from build123d import *

# Parameters (mm, degrees)
SKETCH2_W                                     = 609.6
SKETCH2_H                                     = 914.4
BOSS_EXTRUDE1_DEPTH                           = 25.4
F_1_4_20_TAPPED_HOLE1_D                       = 5.1054
SKETCH46_R                                    = 76.2
CUT_EXTRUDE3_DEPTH                            = 26.4
SKETCH47_R                                    = 50.8
CUT_EXTRUDE4_DEPTH                            = 26.4
CBORE_FOR_1_4_SOCKET_HEAD_CAP_SCREW1_AT_COUNT = 2
CBORE_FOR_1_4_SOCKET_HEAD_CAP_SCREW1_AT_PITCH = 558.8
CBORE_FOR_1_4_SOCKET_HEAD_CAP_SCREW1_2_COUNT  = 2
CBORE_FOR_1_4_SOCKET_HEAD_CAP_SCREW1_2_PITCH  = 1028.621601951
CBORE_FOR_1_4_SOCKET_HEAD_CAP_SCREW1_3_COUNT  = 2
CBORE_FOR_1_4_SOCKET_HEAD_CAP_SCREW1_3_PITCH  = 863.6
CBORE_FOR_1_4_SOCKET_HEAD_CAP_SCREW1_4_COUNT  = 2
CBORE_FOR_1_4_SOCKET_HEAD_CAP_SCREW1_4_PITCH  = 523.634414453
CBORE_FOR_1_4_SOCKET_HEAD_CAP_SCREW1_5_COUNT  = 2
CBORE_FOR_1_4_SOCKET_HEAD_CAP_SCREW1_5_PITCH  = 579.765780294
CBORE_FOR_1_4_SOCKET_HEAD_CAP_SCREW1_6_COUNT  = 2
CBORE_FOR_1_4_SOCKET_HEAD_CAP_SCREW1_6_PITCH  = 452.234142895
CBORE_FOR_1_4_SOCKET_HEAD_CAP_SCREW1_7_COUNT  = 2
CBORE_FOR_1_4_SOCKET_HEAD_CAP_SCREW1_7_PITCH  = 377.598146182


with BuildPart() as part:
    # Sketch2 → Boss-Extrude1 (new body)
    with BuildSketch(Plane(origin=(0, 0, 0), x_dir=(1, 0, 0), z_dir=(0, 1, 0))):
        with Locations((659.0884662, -7.96825605)):
            Rectangle(SKETCH2_W, SKETCH2_H)
    extrude(amount=BOSS_EXTRUDE1_DEPTH)

    # 1/4-20 Tapped Hole1 (through all)
    with Locations(Plane(origin=(0, 25.4, 0), x_dir=(1, 0, 0), z_dir=(0, 1, 0))):
        with Locations((366.9884662, 436.53174395)):
            Hole(F_1_4_20_TAPPED_HOLE1_D / 2)

    # Sketch46 → Cut-Extrude3 (cut, through all)
    with BuildSketch(Plane(origin=(0, 25.4, 0), x_dir=(1, 0, 0), z_dir=(0, 1, 0))):
        with Locations((786.0884662, -261.96825605)):
            Circle(SKETCH46_R)
    extrude(amount=-CUT_EXTRUDE3_DEPTH, mode=Mode.SUBTRACT)

    # Sketch47 → Cut-Extrude4 (cut, through all)
    with BuildSketch(Plane(origin=(0, 25.4, 0), x_dir=(1, 0, 0), z_dir=(0, 1, 0))):
        with Locations((582.8884662, -7.96825605)):
            Circle(SKETCH47_R)
    extrude(amount=-CUT_EXTRUDE4_DEPTH, mode=Mode.SUBTRACT)

    # Sketch51 → CBORE for 1/4 Socket Head Cap Screw1 (revolve, cut)
    with BuildSketch(Plane(origin=(379.6884662, 25.4, -423.83174395), x_dir=(0, 0, 1), z_dir=(1, 0, 0))):
        Polygon((0, 0), (0, 25.4), (3.3782, 25.4), (3.3782, 6.35), (5.55625, 6.35), (5.55625, 0.635), (6.19125, 0), align=None)
    cbore_for_1_4_socket_head_cap_screw1 = revolve(axis=Axis((379.6884662, 31.75, -423.83174395), (0, -1, 0)), mode=Mode.SUBTRACT)

    # CBORE for 1/4 Socket Head Cap Screw1 at: CBORE for 1/4 Socket Head Cap Screw1 ×2
    with Locations(*[(i * CBORE_FOR_1_4_SOCKET_HEAD_CAP_SCREW1_AT_PITCH, 0, 0) for i in range(1, CBORE_FOR_1_4_SOCKET_HEAD_CAP_SCREW1_AT_COUNT)]):
        add(cbore_for_1_4_socket_head_cap_screw1, mode=Mode.SUBTRACT)

    # CBORE for 1_4 Socket Head Cap Screw1 2: CBORE for 1/4 Socket Head Cap Screw1 ×2
    with Locations(*[Vector(0.543251278, 0, 0.839570157) * (i * CBORE_FOR_1_4_SOCKET_HEAD_CAP_SCREW1_2_PITCH) for i in range(1, CBORE_FOR_1_4_SOCKET_HEAD_CAP_SCREW1_2_COUNT)]):
        add(cbore_for_1_4_socket_head_cap_screw1, mode=Mode.SUBTRACT)

    # CBORE for 1_4 Socket Head Cap Screw1 3: CBORE for 1/4 Socket Head Cap Screw1 ×2
    with Locations(*[(0, 0, i * CBORE_FOR_1_4_SOCKET_HEAD_CAP_SCREW1_3_PITCH) for i in range(1, CBORE_FOR_1_4_SOCKET_HEAD_CAP_SCREW1_3_COUNT)]):
        add(cbore_for_1_4_socket_head_cap_screw1, mode=Mode.SUBTRACT)

    # CBORE for 1_4 Socket Head Cap Screw1 4: CBORE for 1/4 Socket Head Cap Screw1 ×2
    with Locations(*[Vector(0.242535625, 0, 0.9701425) * (i * CBORE_FOR_1_4_SOCKET_HEAD_CAP_SCREW1_4_PITCH) for i in range(1, CBORE_FOR_1_4_SOCKET_HEAD_CAP_SCREW1_4_COUNT)]):
        add(cbore_for_1_4_socket_head_cap_screw1, mode=Mode.SUBTRACT)

    # CBORE for 1_4 Socket Head Cap Screw1 5: CBORE for 1/4 Socket Head Cap Screw1 ×2
    with Locations(*[Vector(0.48191875, 0, 0.876215909) * (i * CBORE_FOR_1_4_SOCKET_HEAD_CAP_SCREW1_5_PITCH) for i in range(1, CBORE_FOR_1_4_SOCKET_HEAD_CAP_SCREW1_5_COUNT)]):
        add(cbore_for_1_4_socket_head_cap_screw1, mode=Mode.SUBTRACT)

    # CBORE for 1_4 Socket Head Cap Screw1 6: CBORE for 1/4 Socket Head Cap Screw1 ×2
    with Locations(*[Vector(0.617821552, 0, 0.786318339) * (i * CBORE_FOR_1_4_SOCKET_HEAD_CAP_SCREW1_6_PITCH) for i in range(1, CBORE_FOR_1_4_SOCKET_HEAD_CAP_SCREW1_6_COUNT)]):
        add(cbore_for_1_4_socket_head_cap_screw1, mode=Mode.SUBTRACT)

    # CBORE for 1_4 Socket Head Cap Screw1 7: CBORE for 1/4 Socket Head Cap Screw1 ×2
    with Locations(*[Vector(0.336336397, 0, 0.941741912) * (i * CBORE_FOR_1_4_SOCKET_HEAD_CAP_SCREW1_7_PITCH) for i in range(1, CBORE_FOR_1_4_SOCKET_HEAD_CAP_SCREW1_7_COUNT)]):
        add(cbore_for_1_4_socket_head_cap_screw1, mode=Mode.SUBTRACT)


solid = part.part
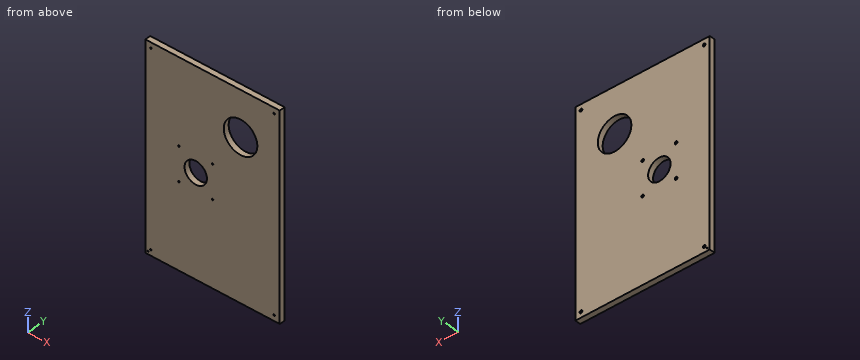
Can you work these out from the model? Positions are in its coordinate system, mm. Round coordinates to 2 decimals unless told otherwise and drop trailing zeros. Order: outer loops, then holes, each group sorted by start corner. A loop starts at its lowest first (then second) coordinate and runs counter-clockwise, first axis right, second up. Notation, with made-up numbers: (74.25, -34) - (89.25, -34) arc R20 ccw to (89.25, -22) - close; hole circle Ø5 at (50, -26.5). An arc over 180 degrees is marked (long way). Answer in a Markdown table with one row per item.
(1) Suppose I cut it at A-A, the plane z = 47. Please give me the cut outline in (x, y), plus the area to 3 significant figures.
From the geometry:
| item | result |
|---|---|
| outline | (354.29, 0) - (550.37, 0) - (550.37, 25.4) - (354.29, 25.4) - close; (615.4, 0) - (963.89, 0) - (963.89, 25.4) - (615.4, 25.4) - close |
| area | 13,800 mm2 |
(2) For P1, Ø5.5, axis at x = 939, z = 438, coming from the +Y side, with a flat end and sliding along its axis, tell me the tip position at first contact or that it passes through.
From the geometry:
| item | result |
|---|---|
| P1 | stops at y = 19.05 |
(3) Suppose I cut it at C-C, the plane y = 10.75. Count the separate pieces of the cut face and the enclosed holes in it, plus the area to 3 significant figures.
From the geometry:
| item | result |
|---|---|
| separate pieces | 1 |
| enclosed holes | 11 |
| area | 531,000 mm2 |
(4) Suppose I cut it at B-B, the plane x = 580. Please give me the cut outline in (y, z).
From the geometry:
| item | result |
|---|---|
| outline | (0, -449.23) - (25.4, -449.23) - (25.4, -42.75) - (0, -42.75) - close; (0, 58.69) - (25.4, 58.69) - (25.4, 465.17) - (0, 465.17) - close |
(5) Please list where these lines run through material, in increasing order: L1, parallel to X at y = 11, z = 82.5; L2, parallel to Z at x = 735, y = 19.75; L3, parallel to Z at x = 792, y = 20. Write a range as from..to.
From the geometry:
| item | result |
|---|---|
| L1 | x = 354.29..503.75, 509.63..656.15, 662.03..963.89 |
| L2 | z = -449.23..205.43, 318.51..465.17 |
| L3 | z = -449.23..186, 337.94..465.17 |
